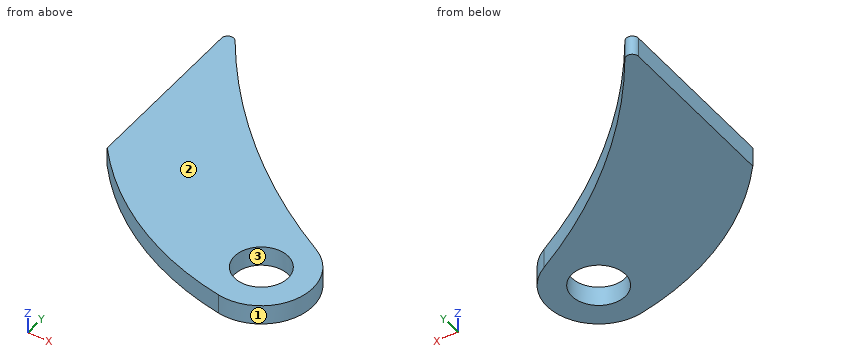
```python
from build123d import *

# Parameters (mm, degrees)
CROQUIS1_R              = 13
SALIENTE_EXTRUIR1_DEPTH = 4.765
REDONDEO2_R             = 3


with BuildPart() as part:
    # Croquis1 → Saliente-Extruir1 (new, symmetric)
    with BuildSketch(Plane.XY):
        with BuildLine():
            Line((-44.5526077, 70.070188004), (-44.5526077, -24.929811996))
            ThreePointArc((-44.5526077, -24.929811996), (-4.556794057, -60.38146366), (45.329796291, -79.559910369))
            ThreePointArc((45.329796291, -79.559910369), (73.459258652, -63.640786047), (62.376657562, -33.278620035))
            ThreePointArc((62.376657562, -33.278620035), (2.406760274, 11.66514835), (-44.5526077, 70.070188004))
        make_face()
        with Locations((50, -55)):
            Circle(CROQUIS1_R, mode=Mode.SUBTRACT)
    extrude(amount=SALIENTE_EXTRUIR1_DEPTH, both=True)

    # Redondeo2
    redondeo2_edges = [part.edges().sort_by_distance(p)[0] for p in [
        (-44.5526077, 70.070188004, 0),
    ]]
    fillet(redondeo2_edges, radius=REDONDEO2_R)


solid = part.part
```
Could you check a few things on this model? Use its own coordinates, in mm. Face numbers are marked on the shaded views. Round coordinates to 2 decimals unless told otherwise and drop trailing zeros. Write each loop counter-clockwise with the first axis right and the second up, starting at its lowest first coordinate (ties: lowest second). Pieces come first, ordered by that corner, then holes. Notation, with made-up numbers: M 33,-36.75 L 43,-36.75 A15 ccw 43,-21.75 Z; hole C 64,70.25 d6. An arc over 180 degrees is marked long. Write each question's results on one line, items separated by ' | '. Start each with the question number.
1. Imagine slicing it at B-B on z = -0.25. List the corners of the cut face in (x, y) for me, and give its area (3 significant figures).
2. Imagine slicing it at D-D on y = 31. List the corners of the cut face in (x, z) for me (3 decimals), and give its area (3 significant figures).
3. I need wall thicknesses on L1, parallel to Y at x = 50, z = 0; L2, parallel to Y at x = 41, z = 1.75; L3, parallel to Y at x = -5.5, z = -2.5. Which ranges of each line are inside material? Lowest first, please. Write a range as from..to.
4. Imagine slicing it at C-C on x = 54.5. List the corners of the cut face in (y, z) for me (3 decimals).
5. I'm going to push flat-ended pins straight in: pin 1 Ø1 at (y, z) = (-35, 0) entering from -X; pin 2 Ø5 at (x, z) = (60.5, 2) entering from +Y. Where does each tip first touch, or does it pass through?
6. Imagine slicing it at A-A on y = -52. List the corners of the cut face in (x, z) for me (3 decimals).
7. Thinking about a two-plate mould opening in Y: for the marked faces 1, 2 and 3, which applies, +Y half, -Y half, draft (parallel to the pull), parting line (faces both ways), or undercut?
Result sheet:
1) outline: M -44.55,-24.93 A150 ccw 45.33,-79.56 A25 ccw 62.38,-33.28 A300 cw -39.05,61.47 A3 ccw -44.55,59.81 Z; hole C 50,-55 d26 | area: 7,590 mm^2
2) outline: M -44.553,-4.765 L -15.898,-4.765 L -15.898,4.765 L -44.553,4.765 Z | area: 273 mm^2
3) L1: y = -80..-68, -42..-25.83 | L2: y = -78.67..-64.38, -45.62..-19.88 | L3: y = -59.8..19.6
4) outline: M -79.592,-4.765 L -67.196,-4.765 L -67.196,4.765 L -79.592,4.765 Z; M -42.804,-4.765 L -28.63,-4.765 L -28.63,4.765 L -42.804,4.765 Z
5) pin 1: stops at x = -36.35 | pin 2: stops at y = -30.74
6) outline: M -16.916,-4.765 L 37.351,-4.765 L 37.351,4.765 L -16.916,4.765 Z; M 62.649,-4.765 L 74.819,-4.765 L 74.819,4.765 L 62.649,4.765 Z
7) face 1: parting line | face 2: draft | face 3: undercut
